Autodesk Inventor part; units mm, degrees
ref_plane "YZ Plane" through (0, 0, 0) normal (1, 0, 0) x (0, 1, 0)
ref_plane "XZ Plane" through (0, 0, 0) normal (0, 1, 0) x (-1, 0, 0)
ref_plane "XY Plane" through (0, 0, 0) normal (0, 0, 1) x (1, 0, 0)
sketch "Sketch1" plane through (0, 0, 0) normal (0, 0, 1) x (1, 0, 0)
  circle A0 centre (0, 0) radius 10
  dimension "d0" = 20
extrude "Extrusion1" add sketch "Sketch1" along normal blind 17.3
sketch "Sketch2" plane through (0, 0, 17.3) normal (0, 0, 1) x (1, 0, 0)
  line L0 (0, 0) -> (0, 7.5)
  circle A0 centre (0, 7.5) radius 1.25
  line L1 (0, 0) -> (0, -7.5)
  circle A1 centre (0, -7.5) radius 1.25
  dimension "d3" = 7.5
  dimension "d4" = 2.5
  dimension "d5" = 7.5
  dimension "d6" = 2.5
extrude "Extrusion2" cut sketch "Sketch2" against normal blind 1
sketch "Sketch3" plane through (0, 0, 17.3) normal (0, 0, 1) x (1, 0, 0)
  circle A0 centre (0, 0) radius 3
  dimension "d9" = 6
extrude "Extrusion3" add sketch "Sketch3" along normal blind 3
sketch "Sketch4" plane through (0, 0, 20.3) normal (0, 0, 1) x (1, 0, 0)
  circle A0 centre (0, 0) radius 2
  dimension "d12" = 4
extrude "Extrusion4" add sketch "Sketch4" along normal blind 14.5
sketch "Sketch5" plane through (0, 0, 34.8) normal (0, 0, 1) x (1, 0, 0)
  line L0 (0, 0) -> (2, 0)
  line L1 (2, 0) -> (1.5, 0)
  circle A0 centre (0, 0) radius 2
  line L2 (1.5, 0) -> (1.5, 1.3229)
  line L3 (1.5, 0) -> (1.5, -1.3229)
  circle A1 centre (0, 0) radius 2
  dimension "d17" = 4
  dimension "d15" = 2
  dimension "d16" = 0.5
extrude "Extrusion5" cut sketch "Sketch5" against normal blind 12.2 contours L2 A0 L0 | L0 A0 L3
sketch "Sketch7" plane through (0, 0, 0) normal (1, 0, 0) x (0, 1, 0)
  line L0 (10, 0) -> (-10, 0)
  line L1 (0, 0) -> (9, 0)
  line L2 (10, -1) -> (10, -25)
  line L3 (10, -25) -> (0, -25)
  line L4 (0, -25) -> (0, 0)
  arc A0 (10, -1) -> (9, 0) centre (9, -1) ccw
  line L5 (0, -25) -> (0, -28)
  line L6 (0, -28) -> (3, -28)
  line L7 (3, -28) -> (4.7321, -25)
  dimension "d20" = 10
  dimension "d21" = 25
  dimension "d22" = 1
  dimension "d23" = 3
  dimension "d24" = 3
  dimension "d25" = 120
revolve "Revolution1" add sketch "Sketch7" angle 360 about axis through (0, 0, -25) along (0, 0, 1)
sketch "Sketch8" plane through (0, 0, 0) normal (1, 0, 0) x (0, 1, 0)
  line L0 (-4.7321, -25) -> (4.7321, -25)
  line L1 (0, -25) -> (8, -25)
  line L2 (8, -25) -> (8, -29.5)
  line L3 (7.5, -30) -> (6.5, -30)
  line L4 (6, -29.5) -> (6, -25)
  arc A0 (7.5, -30) -> (8, -29.5) centre (7.5, -29.5) ccw
  arc A1 (6, -29.5) -> (6.5, -30) centre (6.5, -29.5) ccw
  line L5 (-10, -25) -> (10, -25)
  line L6 (7, -25) -> (7, -29)
  circle A2 centre (7, -29) radius 0.5
  line L7 (0, -25) -> (0, -32)
  line L8 (0, -25) -> (-8, -25)
  line L9 (-8, -25) -> (-8, -29.5)
  line L10 (-7.5, -30) -> (-6.5, -30)
  line L11 (-6, -29.5) -> (-6, -25)
  arc A3 (-8, -29.5) -> (-7.5, -30) centre (-7.5, -29.5) ccw
  arc A4 (-6.5, -30) -> (-6, -29.5) centre (-6.5, -29.5) ccw
  line L12 (-7, -25) -> (-7, -29)
  circle A5 centre (-7, -29) radius 0.5
  point P0 (0, 0)
  point P1 (8, -30)
  point P2 (6, -30)
  point P3 (-8, -30)
  point P4 (-6, -30)
  point P5 (-8, -25)
  point P6 (-6, -25)
  dimension "d27" = 8
  dimension "d28" = 5
  dimension "d29" = 2
  dimension "d30" = 0.5
  dimension "d31" = 4
  dimension "d32" = 1
  dimension "d33" = 7
extrude "Extrusion6" add sketch "Sketch8" along normal mid plane 0.5
properties part number "motor_dc_20d_12v"
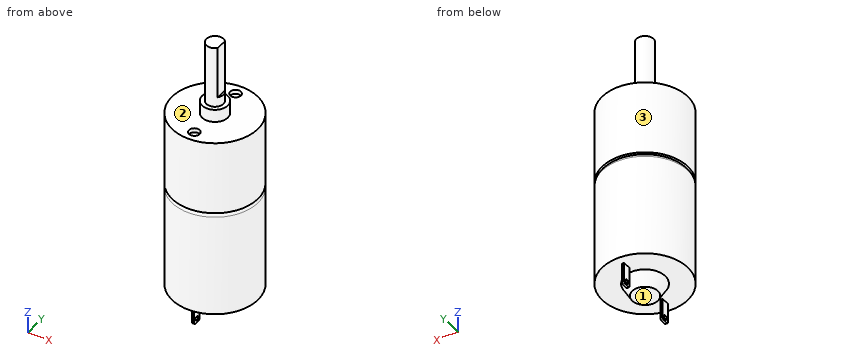
Part model, mm, in its own coordinate system. Face numbers are marked on the shaded views. A direction names the side the tool comes from. Round coordinates to 2 decimals unless told otherwise and drop trailing zeros. Loops run counter-clockwise (first coordinate to the right, second up) from the corner with the lowest first, then second, coordinate; pieces in that order, holes last.
1. Slice it at C-C (z = 23.5). Give the cut face in (x, y).
Solutions:
outline: (1.5, -1.32) - (1.5, 1.32) arc R2 ccw (long way) to start
2. Slice it at A-A (y = 0). Give the cut face in (x, z), and give its area (3 significant figures).
Solutions:
outline: (-10, -25) - (-4.73, -25) - (-3, -28) - (3, -28) - (4.73, -25) - (10, -25) - (10, -1) arc R1 ccw to (9, 0) - (10, 0) - (10, 17.3) - (3, 17.3) - (3, 20.3) - (2, 20.3) - (2, 22.6) - (1.5, 22.6) - (1.5, 34.8) - (-2, 34.8) - (-2, 20.3) - (-3, 20.3) - (-3, 17.3) - (-10, 17.3) - (-10, 0) - (-9, 0) arc R1 ccw to (-10, -1) - close
area: 939 mm2
3. Flat gauge pins, fed straight in: pin 1 (8 mm diameter, centred on x = 7, z = 8, fed in from -Y); pin 2 (1.6 mm diameter, centred on y = -6.5, z = -27, fed in from +X); pin 3 (12 mm diameter, centred on x = 4, z = -13.5, fed in from -Y); pin 4 (1.3 mm diameter, centred on y = 0, z = 30, fed in from +X). Where does each tip first touch, or does it go through?
Solutions:
pin 1: stops at y = -9.54
pin 2: stops at x = 0.25
pin 3: stops at y = -10
pin 4: stops at x = 1.5
4. Drill centre lines: line 1 along Y through (x, z) = (-0.05, -29); line 2 along Y through (x, z) = (0, 16.55); line 3 along Z through (x, y) = (0.15, 7). Where is each one in solid material? Low to high.
Solutions:
line 1: y = -8 to -7.5, -6.5 to -6, 6 to 6.5, 7.5 to 8
line 2: y = -10 to -8.75, -6.25 to 6.25, 8.75 to 10
line 3: z = -30 to -29.5, -28.5 to 16.3
5. 3-axis set-ups, long thin cutter, end or side, ignore diameter. For the marked faces 1, 2 and 3: which of +Z, -Z, +X, -X, +Y, -Y reach the whole face in a straight line?
Solutions:
face 1: -Z, +X, -X
face 2: +Z
face 3: +Z, -Z
6. Slice it at B-B (z = -23). Give the cut face in (x, y), and give its area (3 significant figures).
Solutions:
outline: circle Ø20 at (0, 0)
area: 314 mm2
